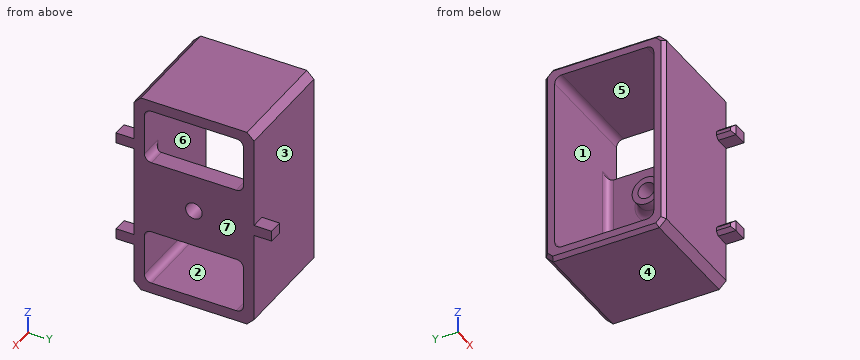
```python
from build123d import *

# Parameters (mm, degrees)
SKETCH2_W             = 14.732
SKETCH2_H             = 8.636
SKETCH2_W_2           = 13.208
SKETCH2_H_2           = 7.112
EXTRUDE_THIN1_DEPTH   = 7.9375
SKETCH3_W             = 14.732
SKETCH3_H             = 8.636
BOSS_EXTRUDE1_DEPTH   = 1.27
CUT_EXTRUDE1_REACH    = 9.938
SKETCH4_W             = 3.949
SKETCH4_H             = 7.112
SKETCH7_R             = 1.016
BOSS_EXTRUDE2_DEPTH   = 1.27
F_0_80_TAPPED_HOLE1_D = 1.19126
SKETCH9_W             = 0.762
SKETCH9_H             = 1.27
EXTRUDE_THIN2_DEPTH   = 1.27
FILLET1_R             = 0.508
CHAMFER1_SIZE         = 0.508
CHAMFER2_SIZE         = 0.254


with BuildPart() as part:
    # Sketch2 → Extrude-Thin1 (new body)
    with BuildSketch(Plane(origin=(-2.794, 0, 0), x_dir=(0, 0, -1), z_dir=(1, 0, 0))):
        with Locations((-7.366, -62.992)):
            Rectangle(SKETCH2_W, SKETCH2_H)
        with Locations((-7.366, -62.992)):
            Rectangle(SKETCH2_W_2, SKETCH2_H_2, mode=Mode.SUBTRACT)
    extrude(amount=EXTRUDE_THIN1_DEPTH)

    # Sketch3 → Boss-Extrude1 (add)
    with BuildSketch(Plane(origin=(5.1435, 0, 0), x_dir=(0, 0, -1), z_dir=(1, 0, 0))):
        with Locations((-7.366, -62.992)):
            Rectangle(SKETCH3_W, SKETCH3_H)
    extrude(amount=-BOSS_EXTRUDE1_DEPTH)

    # Sketch4 → Cut-Extrude1 (cut, up to next)
    with BuildSketch(Plane(origin=(5.1435, 0, 0), x_dir=(0, 0, -1), z_dir=(1, 0, 0)), mode=Mode.PRIVATE) as cut_extrude1_sk1:
        with Locations((-2.7365, -62.992)):
            Rectangle(SKETCH4_W, SKETCH4_H)
    cut_extrude1_tool1 = extrude(cut_extrude1_sk1.sketch, amount=-CUT_EXTRUDE1_REACH, mode=Mode.PRIVATE) & part.part
    add(cut_extrude1_tool1.solids().sort_by_distance((5.1435, -62.992, 2.7365))[0], mode=Mode.SUBTRACT)
    # Sketch4 → Cut-Extrude1 (cut, up to next)
    with BuildSketch(Plane(origin=(5.1435, 0, 0), x_dir=(0, 0, -1), z_dir=(1, 0, 0)), mode=Mode.PRIVATE) as cut_extrude1_sk2:
        with Locations((-11.9955, -62.992)):
            Rectangle(SKETCH4_W, SKETCH4_H)
    cut_extrude1_tool2 = extrude(cut_extrude1_sk2.sketch, amount=-CUT_EXTRUDE1_REACH, mode=Mode.PRIVATE) & part.part
    add(cut_extrude1_tool2.solids().sort_by_distance((5.1435, -62.992, 11.9955))[0], mode=Mode.SUBTRACT)

    # Sketch7 → Boss-Extrude2 (add)
    with BuildSketch(Plane.ZY.offset(-3.8735)):
        with Locations((7.366, -62.992)):
            Circle(SKETCH7_R)
    extrude(amount=BOSS_EXTRUDE2_DEPTH)

    # #0-80 Tapped Hole1 (through all)
    with Locations(Plane(origin=(5.1435, 0, 0), x_dir=(0, 0, -1), z_dir=(1, 0, 0))):
        with Locations((-7.366, -62.992)):
            Hole(F_0_80_TAPPED_HOLE1_D / 2)

    # Sketch9 → Extrude-Thin2 (add)
    with BuildSketch(Plane(origin=(5.1435, 0, 0), x_dir=(0, 0, -1), z_dir=(1, 0, 0))):
        with Locations((-7.366, -58.039)):
            Rectangle(SKETCH9_W, SKETCH9_H)
        with Locations((-11.049, -67.945)):
            Rectangle(SKETCH9_W, SKETCH9_H)
        with Locations((-3.683, -67.945)):
            Rectangle(SKETCH9_W, SKETCH9_H)
    extrude(amount=-EXTRUDE_THIN2_DEPTH)

    # Fillet1
    fillet1_edges = [part.edges().sort_by_distance(p)[0] for p in [
        (3.8735, -66.548, 7.366),
        (1.17475, -59.436, 13.97),
        (1.17475, -59.436, 0.762),
        (1.17475, -66.548, 0.762),
        (3.8735, -59.436, 7.366),
        (1.17475, -66.548, 13.97),
        (4.5085, -59.436, 10.021),
        (4.5085, -59.436, 4.711),
        (4.5085, -66.548, 4.711),
        (4.5085, -66.548, 10.021),
        (3.8735, -62.992, 6.35),
    ]]
    fillet(fillet1_edges, radius=FILLET1_R)

    # Chamfer1
    chamfer1_edges = [part.edges().sort_by_distance(p)[0] for p in [
        (1.17475, -67.31, 14.732),
        (1.17475, -67.31, 0),
        (1.17475, -58.674, 0),
        (1.17475, -58.674, 14.732),
    ]]
    chamfer(chamfer1_edges, length=CHAMFER1_SIZE)

    # Chamfer2
    chamfer2_edges = [part.edges().sort_by_distance(p)[0] for p in [
        (-2.794, -67.056, 14.478),
        (-2.794, -67.31, 7.366),
        (-2.794, -67.056, 0.254),
        (-2.794, -62.992, 0),
        (-2.794, -58.928, 0.254),
        (-2.794, -62.992, 14.732),
        (-2.794, -58.928, 14.478),
        (-2.794, -58.674, 7.366),
        (3.8735, -58.039, 6.985),
        (3.8735, -57.404, 7.366),
        (3.8735, -58.039, 7.747),
        (3.8735, -67.945, 10.668),
        (3.8735, -68.58, 11.049),
        (3.8735, -67.945, 11.43),
        (3.8735, -67.945, 3.302),
        (3.8735, -68.58, 3.683),
        (3.8735, -67.945, 4.064),
    ]]
    chamfer(chamfer2_edges, length=CHAMFER2_SIZE)


solid = part.part
```
CAD build for the part. Positions are in the model's coordinates, mm. Face numbers are marked on the shaded views. A direction names the side the tool comes from. Coordinates: 2 decimals unless noted, no trailing zeros. Order: outer loops, then holes, each group sorted by start corner. A loop starts at its lowest first (then second) coordinate and runs counter-clockwise, first axis right, second up.
(1) Saw through at D-D, the plane z = 2.75. Write the cut outline in (x, y).
Solution:
outline: (-2.79, -67.06) - (-2.54, -67.31) - (5.14, -67.31) - (5.14, -66.55) - (-2.79, -66.55) - close; (-2.79, -59.44) - (5.14, -59.44) - (5.14, -58.67) - (-2.54, -58.67) - (-2.79, -58.93) - close
(2) Mould opens along Z. For the marked faces 1, 2, 3 and 4 say: released by +Z, released by -Z, zero draft, split by the parting line, or undercut.
Solution:
face 1: undercut
face 2: undercut
face 3: zero draft
face 4: released by -Z
(3) Pin check, flat tips, straight feed: pin 1 Ø0.5 at (x, y) = (4.5, -58.5) entering from +Z; pin 2 Ø2.5 at (x, z) = (2, 9.5) entering from -Y; pin 3 Ø0.5 at (x, y) = (4.5, -68) entering from +Z. Stop position of each tip, or through.
Solution:
pin 1: stops at z = 14.3
pin 2: stops at y = -67.31
pin 3: stops at z = 11.43
(4) Saw through at A-A, the plane y = -60.25. Write the cut outline in (x, z).
Solution:
outline: (-2.79, 0.25) - (-2.54, 0) - (5.14, 0) - (5.14, 0.76) - (-2.79, 0.76) - close; (-2.79, 13.97) - (5.14, 13.97) - (5.14, 14.73) - (-2.54, 14.73) - (-2.79, 14.48) - close; (3.87, 4.71) - (5.14, 4.71) - (5.14, 10.02) - (3.87, 10.02) - close
(5) Which spindle directions (+Z, -Z, +X, -X, +Y, -Y) get a long thin tool onto all of the face, cutting with end or side? Do the marked faces 5, 6 and 7. Say none if no direction does.
Solution:
face 5: +X, -X
face 6: -X
face 7: +Z, -Z, +X, +Y, -Y
(6) Saw through at C-C, the plane z = 4.5. Write the cut outline in (x, y), and give its area (3 significant figures).
Solution:
outline: (-2.79, -67.06) - (-2.54, -67.31) - (5.14, -67.31) - (5.14, -66.45) - (3.66, -66.45) arc R0.51 cw to (3.37, -66.55) - (-2.79, -66.55) - close; (-2.79, -59.44) - (3.37, -59.44) arc R0.51 cw to (3.66, -59.53) - (5.14, -59.53) - (5.14, -58.67) - (-2.54, -58.67) - (-2.79, -58.93) - close
area: 12.3 mm2
(7) Saw through at B-B, the plane x = 1.75. Write the cut outline in (y, z), and give its area (3 significant figures).
Solution:
outline: (-67.31, 0.51) - (-66.8, 0) - (-59.18, 0) - (-58.67, 0.51) - (-58.67, 14.22) - (-59.18, 14.73) - (-66.8, 14.73) - (-67.31, 14.22) - close; hole (-66.55, 1.27) arc R0.51 ccw to (-66.04, 0.76) - (-59.94, 0.76) arc R0.51 ccw to (-59.44, 1.27) - (-59.44, 13.46) arc R0.51 ccw to (-59.94, 13.97) - (-66.04, 13.97) arc R0.51 ccw to (-66.55, 13.46) - close
area: 33.0 mm2
(8) Drill centre lines: L1, parallel to Y at x = -2.5, z = 4.5; L2, parallel to Z at x = -1.25, y = -65; L3, parallel to Y at x = 3.75, z = 7.5. Where is each one in solid material? Low to high.
Solution:
L1: y = -67.31 to -66.55, -59.44 to -58.67
L2: z = 0 to 0.76, 13.97 to 14.73
L3: y = -67.31 to -66.37, -64.18 to -63.57, -62.41 to -61.81, -59.61 to -58.67
